from build123d import *

# Parameters (mm, degrees)
BASE_SKETCH_W   = 33
BASE_SKETCH_H   = 33.5
BASE_DEPTH      = 25
DRILL_SKETCH_R  = 2.25
DRILL_DEPTH     = 45.938847337
MILL_START      = -4.5
MILL_SKETCH_W   = 7.5
MILL_SKETCH_H   = 4.5
MILL_DEPTH      = 4.5
C_BORE_START    = -4.5
C_BORE_SKETCH_R = 3.75
C_BORE_DEPTH    = 4.5


with BuildPart() as part:
    # Base_Sketch → Base (new body)
    with BuildSketch(Plane.XY):
        with Locations((0, 16.75)):
            Rectangle(BASE_SKETCH_W, BASE_SKETCH_H)
    extrude(amount=-BASE_DEPTH)

    # Drill_Sketch → Drill (cut, through all)
    with BuildSketch(Plane.XY):
        with Locations((0, 4.5)):
            Circle(DRILL_SKETCH_R)
        with Locations((-8, 14.5)):
            Circle(DRILL_SKETCH_R)
        with Locations((8, 14.5)):
            Circle(DRILL_SKETCH_R)
    extrude(amount=-DRILL_DEPTH, mode=Mode.SUBTRACT)

    # Mill_Sketch → Mill (cut)
    with BuildSketch(Plane.XY.offset(MILL_START)):
        with Locations((0, 2.25)):
            Rectangle(MILL_SKETCH_W, MILL_SKETCH_H)
    extrude(amount=MILL_DEPTH, mode=Mode.SUBTRACT)

    # C_Bore_Sketch → C_Bore (cut)
    with BuildSketch(Plane.XY.offset(C_BORE_START)):
        with Locations((-8, 14.5)):
            Circle(C_BORE_SKETCH_R)
        with Locations((8, 14.5)):
            Circle(C_BORE_SKETCH_R)
        with Locations((0, 4.5)):
            Circle(C_BORE_SKETCH_R)
    extrude(amount=C_BORE_DEPTH, mode=Mode.SUBTRACT)


solid = part.part
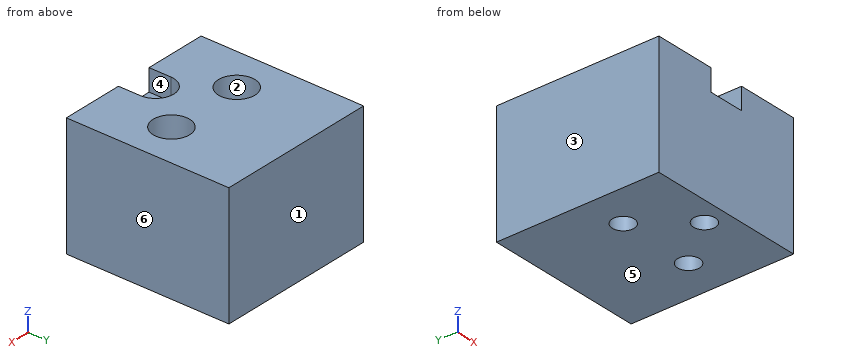
For this review, take the finished solid that the model builds, in its own axes (mm). Face numbers are marked on the shaded views. A direction names the side the tool comes from. Coordinates: 2 decimals unless noted, no trailing zeros. Loops run counter-clockwise (first coordinate to the right, second up) from the corner with the lowest first, then second, coordinate; pieces in that order, holes last. Notation, with made-up numbers: (-1, 86) - (11, 86) arc R25 ccw to (11, 112) - close; hole circle Ø8 at (58, 57). An arc over 180 degrees is marked (long way). Use a Markdown table: item, result. Add a question column.
Item 1: For line 1 (X direction, y = 4.5, z = -20.5); line 2 (Y direction, x = -8, z = -17.5); line 3 (Y direction, x = 8, z = -2.95), list the stretches that pass through material, from the lowest coordinate up.
Item 2: We need section C-C (z = -22). Give the boundary of the cut face in (x, y).
Item 3: Tool access review of the marked faces 1 and 2: name each direction out of +Z, -Z, +X, -X, +Y, -Y from which nothing blocks a thin tool from reaching the whole face with its end or side.
Item 4: We need section A-A (x = 0). Give the boundary of the cut face in (y, z), and give its area (3 significant figures).
Item 5: We need section B-B (y = 14.5). Give the boundary of the cut face in (x, z).
Item 6: Insertion check: pin 1 Ø2 at (x, y) = (8.5, 13) entering from +Z. The pin has a flat end and moves straight along its axis. Give the tip position at first contact, or say it passes through.
Item 7: We need section D-D (x = 11). Give the boundary of the cut face in (y, z).
Item 8: Mouldability with a two-part tool opening along X and no side actions: class the marked faces 3, 4, 5 and 6 as pulls with the +X half, pulls with the -X half, needs draft (parallel to the pull), parting line crosses it, or undercut.
Results list:
| question | item | result |
|---|---|---|
| 1 | line 1 | x = -16.5 to -2.25, 2.25 to 16.5 |
| 1 | line 2 | y = 0 to 12.25, 16.75 to 33.5 |
| 1 | line 3 | y = 0 to 10.75, 18.25 to 33.5 |
| 2 | outline | (-16.5, 0) - (16.5, 0) - (16.5, 33.5) - (-16.5, 33.5) - close; hole circle Ø4.5 at (-8, 14.5); hole circle Ø4.5 at (0, 4.5); hole circle Ø4.5 at (8, 14.5) |
| 3 | face 1 | +Z, -Z, +X, -X, +Y |
| 3 | face 2 | +Z |
| 4 | outline | (0, -25) - (2.25, -25) - (2.25, -4.5) - (0, -4.5) - close; (6.75, -25) - (33.5, -25) - (33.5, 0) - (8.25, 0) - (8.25, -4.5) - (6.75, -4.5) - close |
| 4 | area | 708 mm^2 |
| 5 | outline | (-16.5, -25) - (-10.25, -25) - (-10.25, -4.5) - (-11.75, -4.5) - (-11.75, 0) - (-16.5, 0) - close; (-5.75, -25) - (5.75, -25) - (5.75, -4.5) - (4.25, -4.5) - (4.25, 0) - (-4.25, 0) - (-4.25, -4.5) - (-5.75, -4.5) - close; (10.25, -25) - (16.5, -25) - (16.5, 0) - (11.75, 0) - (11.75, -4.5) - (10.25, -4.5) - close |
| 6 | pin 1 | stops at z = -4.5 |
| 7 | outline | (0, -25) - (33.5, -25) - (33.5, 0) - (16.75, 0) - (16.75, -4.5) - (12.25, -4.5) - (12.25, 0) - (0, 0) - close |
| 8 | face 3 | pulls with the -X half |
| 8 | face 4 | undercut |
| 8 | face 5 | needs draft |
| 8 | face 6 | pulls with the +X half |
